Design review of the part built by this model. Coordinates are the model's own, in mm. Face numbers are marked on the shaded views. A direction names the side the tool comes from. Give positions to 0.01 mm unless a question says otherwise; leave off trailing zeros. Loops run counter-clockwise (first coordinate to the right, second up) from the corner with the lowest first, then second, coordinate; pieces in that order, holes last.
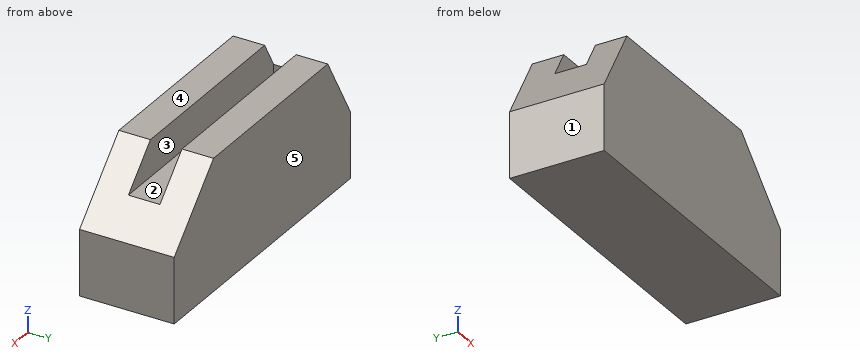
from build123d import *

# Parameters (mm, degrees)
F0_W     = 1422.4
F0_H     = 317.5
F1_DEPTH = 457.2
F2_W     = 73.0727104677
F2_H     = 152.4
F2_W_2   = 207.264
F2_W_3   = 921.5912895323
F3_DEPTH = 177.8


with BuildPart() as f1:
    # F0 (on Front) → F1 (new body)
    with BuildSketch(Plane.XZ):
        with Locations((711.2, 158.75)):
            Rectangle(F0_W, F0_H)
        Polygon((183.3087104677, 635), (0, 317.5), (1422.4, 317.5), (1104.9, 635), align=None)
    extrude(amount=F1_DEPTH)

    # F2 (on face) → F3 (cut)
    with BuildSketch(Plane.XY.offset(635)):
        with Locations((146.7723552339, -228.6)):
            Rectangle(F2_W, F2_H)
        with Locations((1208.532, -228.6)):
            Rectangle(F2_W_2, F2_H)
        with Locations((644.1043552339, -228.6)):
            Rectangle(F2_W_3, F2_H)
    extrude(amount=-F3_DEPTH, mode=Mode.SUBTRACT)


solid = f1.part
Q1. Tool access review of the marked faces 1 and 2: name each direction out of +Z, -Z, +X, -X, +Y, -Y from which nothing blocks a thin tool from reaching the whole face with its end or side.
Results:
face 1: +Z, -Z, -X, +Y, -Y
face 2: +Z, +X
Q2. Insertion check: pin 1 (5 mm diameter, centred on x = 318.5, y = -216.5, fed in from -Z); pin 2 (12 mm diameter, centred on y = -180, z = 400.5, fed in from -X); pin 3 (4 mm diameter, centred on y = -329, z = 385.5, fed in from -X); pin 4 (2 mm diameter, centred on x = 1113, y = -102, fed in from +Z). Each pin has a flat end and moves straight along its axis. Give the tip position at first contact, or say it passes through.
Results:
pin 1: stops at z = 0
pin 2: stops at x = 44.46
pin 3: stops at x = 38.11
pin 4: stops at z = 627.9
Q3. Take a section at C-C (y = -50.5). Give the boundary of the cut face in (x, z).
Results:
outline: (0, 0) - (1422.4, 0) - (1422.4, 317.5) - (1104.9, 635) - (183.31, 635) - (0, 317.5) - close
Q4. Wall thickness on line 1 (Y direction, x = 1244, z = 471); line 2 (Z direction, x = 616, y = -183); line 3 (X direction, y = -272.5, z = 474): over which ranges is each line inside the solid? List them lowest first.
Results:
line 1: y = -457.2 to -304.8, -152.4 to 0
line 2: z = 0 to 457.2
line 3: x = 90.36 to 110.24
Q5. Take a section at B-B (x = 1213). Give the boundary of the cut face in (y, z).
Results:
outline: (-457.2, 0) - (0, 0) - (0, 526.9) - (-152.4, 526.9) - (-152.4, 457.2) - (-304.8, 457.2) - (-304.8, 526.9) - (-457.2, 526.9) - close
Q6. Draft analysis for pull direction Y (two halves, no side actions). For the marked faces 3, 4 and 5, state which applies: pulls with the +Y half, pulls with the -Y half, needs draft (parallel to the pull), parting line crosses it, or undercut.
Results:
face 3: undercut
face 4: needs draft
face 5: pulls with the +Y half
Q7. Take a section at D-D (y = -260.5). Give the boundary of the cut face in (x, z), plus the area to 3 significant figures.
Results:
outline: (0, 0) - (1422.4, 0) - (1422.4, 317.5) - (1282.7, 457.2) - (110.24, 457.2) - (110.24, 508.43) - (0, 317.5) - close
area: 636,000 mm2
Q8. Take a section at A-A (z = 549). Give the boundary of the cut face in (x, y).
Results:
outline: (133.66, -457.2) - (1190.9, -457.2) - (1190.9, -304.8) - (133.66, -304.8) - close; (133.66, -152.4) - (1190.9, -152.4) - (1190.9, 0) - (133.66, 0) - close
